from build123d import *

# Parameters (mm, degrees)
SKETCH_W        = 230
SKETCH_H        = 75
PAD_DEPTH       = 6.2
SKETCH001_W     = 211
SKETCH001_H     = 4
POCKET_DEPTH    = 3.2
CHAMFER_SIZE    = 2
SKETCH002_R     = 2.6
POCKET001_DEPTH = 10
SKETCH003_W     = 47.4
SKETCH003_H     = 27.2
POCKET002_DEPTH = 7
SKETCH004_W     = 15
SKETCH004_H     = 30
POCKET003_DEPTH = 5.6
SKETCH005_W     = 16
SKETCH005_H     = 13.2
POCKET004_DEPTH = 8
SKETCH006_W     = 20.5
SKETCH006_H     = 18.5
POCKET005_DEPTH = 5.6
SKETCH007_W     = 27
SKETCH007_H     = 25
SKETCH007_W_2   = 20.5
SKETCH007_H_2   = 18.5
PAD001_DEPTH    = 20
CHAMFER001_SIZE = 3
SKETCH008_R     = 1.25
POCKET006_DEPTH = 30


with BuildPart() as part:
    # Sketch → Pad (new body)
    with BuildSketch(Plane.XY):
        Rectangle(SKETCH_W, SKETCH_H)
    extrude(amount=PAD_DEPTH)

    # Sketch001 (on Face6 of Pad) → Pocket (cut)
    with BuildSketch(Plane.XY.offset(6.2)):
        with Locations((9.5, 35.5)):
            Rectangle(SKETCH001_W, SKETCH001_H)
    extrude(amount=-POCKET_DEPTH, mode=Mode.SUBTRACT)

    # Chamfer
    chamfer_edges = [part.edges().sort_by_distance(p)[0] for p in [
        (-115, 0, 0),
        (0, -37.5, 0),
        (115, 0, 0),
    ]]
    chamfer(chamfer_edges, length=CHAMFER_SIZE)

    # Sketch002 (on Face4 of Chamfer) → Pocket001 (cut)
    with BuildSketch(Plane.XY.offset(6.2)):
        with Locations((-100, -22.5)):
            Circle(SKETCH002_R)
        with Locations((0, -22.5)):
            Circle(SKETCH002_R)
        with Locations((100, -22.5)):
            Circle(SKETCH002_R)
        with Locations((-100, 22.5)):
            Circle(SKETCH002_R)
    extrude(amount=-POCKET001_DEPTH, mode=Mode.SUBTRACT)

    # Sketch003 (on Face8 of Pocket001) → Pocket002 (cut)
    with BuildSketch(Plane(origin=(0, 0, 0), x_dir=(1, 0, 0), z_dir=(0, 0, -1))):
        with Locations((43.7, -14.6)):
            Rectangle(SKETCH003_W, SKETCH003_H)
    extrude(amount=-POCKET002_DEPTH, mode=Mode.SUBTRACT)

    # Sketch004 (on Face4 of Pocket002) → Pocket003 (cut)
    with BuildSketch(Plane.XY.offset(6.2)):
        with Locations((30.7, 14.6)):
            Rectangle(SKETCH004_W, SKETCH004_H)
        with Locations((56.7, 14.6)):
            Rectangle(SKETCH004_W, SKETCH004_H)
    extrude(amount=-POCKET003_DEPTH, mode=Mode.SUBTRACT)

    # Sketch005 (on Face4 of Pocket003) → Pocket004 (cut)
    with BuildSketch(Plane.XY.offset(6.2)):
        with Locations((-40, 14.2)):
            Rectangle(SKETCH005_W, SKETCH005_H)
    extrude(amount=-POCKET004_DEPTH, mode=Mode.SUBTRACT)

    # Sketch006 (on Face4 of Pocket004) → Pocket005 (cut)
    with BuildSketch(Plane.XY.offset(6.2)):
        with Locations((-40, 14.2)):
            Rectangle(SKETCH006_W, SKETCH006_H)
    extrude(amount=-POCKET005_DEPTH, mode=Mode.SUBTRACT)

    # Sketch007 (on Face4 of Pocket005) → Pad001 (join)
    with BuildSketch(Plane.XY.offset(6.2)):
        with Locations((-40, 14.2)):
            Rectangle(SKETCH007_W, SKETCH007_H)
        with Locations((-40, 14.2)):
            Rectangle(SKETCH007_W_2, SKETCH007_H_2, mode=Mode.SUBTRACT)
    extrude(amount=PAD001_DEPTH)

    # Chamfer001
    chamfer001_edges = [part.edges().sort_by_distance(p)[0] for p in [
        (-53.5, 1.7, 16.2),
        (-26.5, 1.7, 16.2),
        (-53.5, 26.7, 16.2),
        (-26.5, 26.7, 16.2),
    ]]
    chamfer(chamfer001_edges, length=CHAMFER001_SIZE)

    # Sketch008 (on Face5 of Chamfer001) → Pocket006 (cut)
    with BuildSketch(Plane(origin=(-53.5, 0, 0), x_dir=(0, -1, 0), z_dir=(-1, 0, 0))):
        with Locations((-14.2, 16.2)):
            Circle(SKETCH008_R)
    extrude(amount=-POCKET006_DEPTH, mode=Mode.SUBTRACT)


solid = part.part
Work out the finished part from the listing and answer in its coordinate system (mm). A direction names the side the tool comes from. Round coordinates to 2 decimals unless told otherwise and drop trailing zeros. Write each loop counter-clockwise with the first axis right and the second up, starting at its lowest first coordinate (ties: lowest second). Pieces come first, ordered by that corner, then holes.
1) The mould has two halves that part along X. Classify faces 1 (the cylindrical face through (-101.916, -20.743, 3.143)), 2 (the flat face through (-115, -1, 4)), 3 (the flat face through (-2, -37.5, 4)): pulls with the +X half, pulls with the -X half, needs draft (parallel to the pull), parting line crosses it, or undercut.
2) A cutting plane is placed at C-C (z = 11.25). Give the vertices of the cut face in (x, y).
3) A cutting plane is placed at D-D (x = 100). Give the vertices of the cut face in (y, z).
4) A tool of negligible diameter and unlimited length cuts with its end or side. For faces 4 (the flat face through (-53.5, 12, 16)), 5 (the flat face through (-26.5, 12, 16)), 6 (the flat face through (43, 1, 3)), 7 (the flat face through (31, 29.6, 3)), 8 (the flat face through (-2, 37.5, 2)), from which of +Z, -Z, +X, -X, +Y, -Y can it reach the whole face along a straight path? Write none if from no direction.
5) Given pin 1 Ø3 at (y, z) = (14.2, 16.2) entering from -X; pin 2 Ø5.5 at (y, z) = (14, 16.5) entering from +X; pin 3 Ø1.5 at (x, y) = (-62, 15) entering from +Z, each flat-ended and moving along its own axis, determine where each tip first touches the part or whether it passes through.
6) A cutting plane is placed at A-A (x = -100). Give the vertices of the cut face in (y, z).
7) Straight lines are drawn through the part: line 1 (Y direction, x = -100, z = 3.75); line 2 (Z direction, x = -27, y = 14); line 3 (Y direction, x = 100, z = 2). For each, find the intervals that lie inside material, in ascending order.
8) A cutting plane is placed at B-B (y = -22.5). Give the vertices of the cut face in (x, z), plus the area to 3 significant figures.
Completed:
1. face 1: undercut
1. face 2: pulls with the -X half
1. face 3: needs draft
2. outline: (-53.5, 4.7) - (-50.5, 1.7) - (-29.5, 1.7) - (-26.5, 4.7) - (-26.5, 23.7) - (-29.5, 26.7) - (-50.5, 26.7) - (-53.5, 23.7) - close; hole (-50.25, 4.95) - (-29.75, 4.95) - (-29.75, 23.45) - (-50.25, 23.45) - close
3. outline: (-37.5, 2) - (-35.5, 0) - (-25.1, 0) - (-25.1, 6.2) - (-37.5, 6.2) - close; (-19.9, 0) - (37.5, 0) - (37.5, 3) - (33.5, 3) - (33.5, 6.2) - (-19.9, 6.2) - close
4. face 4: +Z, -X, +Y, -Y
4. face 5: +Z, +X, +Y, -Y
4. face 6: +Z, -Z
4. face 7: +Z
4. face 8: +Z, -Z, +X, -X, +Y
5. pin 1: stops at x = -53.5
5. pin 2: stops at x = -26.5
5. pin 3: stops at z = 6.2
6. outline: (-37.5, 2) - (-35.5, 0) - (-25.1, 0) - (-25.1, 6.2) - (-37.5, 6.2) - close; (-19.9, 0) - (19.9, 0) - (19.9, 6.2) - (-19.9, 6.2) - close; (25.1, 0) - (37.5, 0) - (37.5, 6.2) - (25.1, 6.2) - close
7. line 1: y = -37.5 to -25.1, -19.9 to 19.9, 25.1 to 37.5
7. line 2: z = 0 to 14.97, 17.43 to 26.2
7. line 3: y = -37.5 to -25.1, -19.9 to 37.5
8. outline: (-115, 2) - (-113, 0) - (-102.6, 0) - (-102.6, 6.2) - (-115, 6.2) - close; (-97.4, 0) - (-2.6, 0) - (-2.6, 6.2) - (-97.4, 6.2) - close; (2.6, 0) - (97.4, 0) - (97.4, 6.2) - (2.6, 6.2) - close; (102.6, 0) - (113, 0) - (115, 2) - (115, 6.2) - (102.6, 6.2) - close
8. area: 1,330 mm2
